from build123d import *

# Parameters (mm, degrees)
SKETCH1_R              = 3.15
BOSS_EXTRUDE1_DEPTH    = 19.05
CUT_EXTRUDE2_OUTLINE_W = 1.95
CUT_EXTRUDE2_OUTLINE_H = 13.132587


# Read off the part's stored shape, not the designer's step: Cut-Extrude2
with BuildPart() as part:
    # Sketch1 → Boss-Extrude1 (new body)
    with BuildSketch(Plane.XY):
        with BuildLine():
            Line((0, 19.05), (0, 0))
            Line((0, 0), (6.152664584, 0))
            ThreePointArc((6.152664584, 0), (34.921438813, 8.919808212), (6.556238945, 19.05))
            Line((6.556238945, 19.05), (0, 19.05))
        make_face()
        with Locations(Location((19.05, 9.525, 0), (0, 0, 180))):
            Circle(SKETCH1_R, mode=Mode.SUBTRACT)
    extrude(amount=BOSS_EXTRUDE1_DEPTH)

    # Cut-Extrude2 outline → Cut-Extrude2 (revolve, cut)
    with BuildSketch(Plane(origin=(19.05, 0, 9.525), x_dir=(1, 0, 0), z_dir=(0, 0, 1))):
        with Locations((0.975, 18.564815995)):
            Rectangle(CUT_EXTRUDE2_OUTLINE_W, CUT_EXTRUDE2_OUTLINE_H)
    revolve(axis=Axis((19.05, 0, 9.525), (0, 1, 0)), mode=Mode.SUBTRACT)


solid = part.part
Input: part model. Units: mm. Frame: model coordinates. A direction names the side the tool comes from. Coordinates: 2 decimals unless noted, no trailing zeros. Order: outer loops, then holes, each group sorted by start corner. A loop starts at its lowest first (then second) coordinate and runs counter-clockwise, first axis right, second up.
1. Cut plane C-C, the plane z = 3.5. Return loops of the section in (x, y) (3 decimals), plus the area to 3 significant figures.
Checked values:
outline: (0, 0) - (6.153, 0) arc R15.875 ccw (long way) to (6.556, 19.05) - (0, 19.05) - close; hole circle Ø6.3 at (19.05, 9.525)
area: 840 mm2
2. Cut plane D-D, the plane x = 7. Return loops of the section in (y, z), plus the area to 3 significant figures.
Checked values:
outline: (-1.08, 0) - (19.59, 0) - (19.59, 19.05) - (-1.08, 19.05) - close
area: 394 mm2
3. Access query for faces 1 (the flat face through (0, 10, 9)), 2 (the flat face through (3, 19.05, 9)), 3 (the cylindrical face through (18.8, 18.66, 7.59)). Directions: +Z, -Z, +X, -X, +Y, -Y. A direction counts if a zero-diameter tool reaches every point of the face in a straight line with its end or side. Return the directions, or none.
Checked values:
face 1: +Z, -Z, -X, +Y, -Y
face 2: +Z, -Z, -X, +Y
face 3: +Y
4. Draft query along Y for faces 4 (the cylindrical face through (19.46, 6.4, 9.39)), 5 (the cylindrical face through (34.9, 8.4, 9.4)), 6 (the flat face through (3, 0, 9)), 7 (the flat face through (17, 13, 19.05)). Return one class per face: +Y half, -Y half, draft (parallel to the pull), parting line (faces both ways), or undercut.
Checked values:
face 4: undercut
face 5: parting line
face 6: -Y half
face 7: draft
5. Contact query for flat-ended pins moving along their axis: P1, Ø6, axis at y = 4.5, z = 7.5, coming from the +X side; P2, Ø1, axis at x = 8, z = 5.5, coming from the -Y side; P3, Ø2, axis at x = 22.5, z = 13, coming from the +Y side; P4, Ø5.5, axis at x = 19.05, y = 9.525, coming from the -Z side. Output: stop coordinate, or through.
Checked values:
P1: stops at x = 34.83
P2: stops at y = -2.61
P3: stops at y = 24.94
P4: passes through
6. Ray query, line 1 along Y through (x, z) = (19.05, 13) (3 decimals); line 2 along X through (y, z) = (9.5, 16.5); line 3 along Z through (x, y) = (19.05, 19.5) (3 decimals). Return the intervals inside material, ascending.
Checked values:
line 1: y = -6.619 to 6.375, 12.675 to 25.131
line 2: x = 0 to 15.9, 22.2 to 34.92
line 3: z = 0 to 7.575, 11.475 to 19.05
7. Cut plane A-A, the plane x = 19.05. Return loops of the section in (y, z) (3 decimals).
Checked values:
outline: (-6.619, 0) - (6.375, 0) - (6.375, 19.05) - (-6.619, 19.05) - close; (12.675, 0) - (25.131, 0) - (25.131, 7.575) - (12.675, 7.575) - close; (12.675, 11.475) - (25.131, 11.475) - (25.131, 19.05) - (12.675, 19.05) - close
8. Cut plane B-B, the plane y = 22. Return loops of the section in (x, z) (3 decimals).
Checked values:
outline: (9.584, 0) - (28.516, 0) - (28.516, 19.05) - (9.584, 19.05) - close; hole circle Ø3.9 at (19.05, 9.525)
